Autodesk Inventor part; units mm, degrees
ref_plane "YZ Plane" through (0, 0, 0) normal (1, 0, 0) x (0, 1, 0)
ref_plane "XZ Plane" through (0, 0, 0) normal (0, 1, 0) x (-1, 0, 0)
ref_plane "UCS1: YZ Plane" through (-0.5, 0, 50) normal (0.9659, 0, 0.2588) x (0.2588, 0, -0.9659)
sketch "Sketch1" plane through (0, 0, 0) normal (0, 0, 1) x (1, 0, 0)
  circle A0 centre (0, 0) radius 0.5
  dimension "d0" = 1
extrude "Extrusion1" add sketch "Sketch1" along normal blind 50
sketch "Sketch2" plane through (0, 0, 50) normal (0, 0, 1) x (1, 0, 0)
  circle A0 centre (0, 0) radius 0.5
  line L0 (-0.7, 0) -> (0.7, 0)
  line L1 (0, -0.7) -> (0, 0.7)
  point P0 (0, 0.5)
  point P1 (0.5, 0)
  point P2 (-0.5, 0)
sketch "Sketch3" plane through (-0.5, 0, 50) normal (0, 1, 0) x (0.9659, 0, 0.2588)
  point P0 (0, 0)
sketch "Sketch4" plane through (0, 0, 0) normal (0, 1, 0) x (-1, 0, 0)
  line L0 (-0.5, 0) -> (-0.5, 50)
  line L1 (0.5, 0) -> (0.5, 50)
  line L2 (0.5, 50) -> (-0.5, 47.2525)
  line L3 (-0.5, 50) -> (0.5, 50)
  point P0 (0, 0)
  dimension "d9" = 70
extrude "Extrusion2" cut sketch "Sketch4" along normal through all both and the other way through all
sketch "Sketch5" plane through (0, 0, 0) normal (0, 0, -1) x (-1, 0, 0)
  circle A0 centre (0, 0) radius 0.5
  circle A1 centre (0, 0) radius 0.35
  dimension "d12" = 0.7
extrude "Hole" cut sketch "Sketch5" against normal through all contours A1
ref_plane "Work Plane1" through (0, 0, 30) normal (0, 0, 1) x (1, 0, 0)
sketch "Sketch6" plane through (0, 0, 30) normal (0, 0, 1) x (1, 0, 0)
  circle A0 centre (0, 0) radius 0.6
  dimension "d16" = 1.2
extrude "Extrusion4" [suppressed]
properties part number "Needle3" material "Stainless Steel, 440C"
Input: part model. Units: mm. Frame: model coordinates. Coordinates: 2 decimals unless noted, no trailing zeros. Loops run counter-clockwise (first coordinate to the right, second up) from the corner with the lowest first, then second, coordinate; pieces in that order, holes last. Notation, with made-up numbers: (45.25, 75.5) -> (69.25, 75.5) arc R23 ccw to (69.25, 97.5) -> close; hole circle Ø10 at (60, -35). An arc over 180 degrees is marked (long way). One line per item, written item: value.
(1) Ray query, line 1 along X through (y, z) = (0, 30.5); line 2 along Y through (x, z) = (-0.3, 38.5). Return the intervals inside material, ascending.
Answer below:
line 1: x = -0.5 to -0.35, 0.35 to 0.5
line 2: y = -0.4 to -0.18, 0.18 to 0.4
(2) Cut plane A-A (x = 0.1). Output: boundary loops of the cut face in (y, z), then the cut area to 3 significant figures.
Answer below:
outline: (-0.49, 0) -> (-0.34, 0) -> (-0.34, 48.35) -> (-0.49, 48.35) -> close; (0.34, 0) -> (0.49, 0) -> (0.49, 48.35) -> (0.34, 48.35) -> close
area: 14.9 mm2
(3) Cut plane C-C (y = 0). Output: boundary loops of the cut face in (x, z).
Answer below:
outline: (-0.5, 0) -> (-0.35, 0) -> (-0.35, 49.59) -> (-0.5, 50) -> close; (0.35, 0) -> (0.5, 0) -> (0.5, 47.25) -> (0.35, 47.66) -> close
(4) Cut plane B-B (z = 32.5). Output: boundary loops of the cut face in (x, y), then the cut area to 3 significant figures.
Answer below:
outline: circle Ø1 at (0, 0); hole circle Ø0.7 at (0, 0)
area: 0.401 mm2
